```python
from build123d import *


with BuildPart() as part:
    # Sweep5: sweep along a path in Sketch1
    with BuildLine(Plane.XY) as sweep5_path:
        Line((0, 0), (0, 450))
        ThreePointArc((0, 450), (14.644660941, 485.355339059), (50, 500))
        Line((50, 500), (450, 500))
        ThreePointArc((450, 500), (485.355339059, 514.644660941), (500, 550))
        Line((500, 550), (500, 1000))
    # Sketch12 → Sweep5 (sweep)
    with BuildSketch(Plane(origin=(0, 0, 0), x_dir=(1, 0, 0), z_dir=(0, 1, 0))):
        Polygon((-14.43375673, -25), (14.43375673, -25), (28.867513459, 0), (14.43375673, 25), (-14.43375673, 25), (-28.867513459, 0), align=None)
    sweep(path=sweep5_path.line)


solid = part.part
```
Geometry check sheet. Reference: the model listing, model coordinates, mm. A direction names the side the tool comes from. Coordinates: 2 decimals unless noted, no trailing zeros. Order: outer loops, then holes, each group sorted by start corner. A loop starts at its lowest first (then second) coordinate and runs counter-clockwise, first axis right, second up.
Q1. Sectioned sample at B-B on z = -15. Record the cut outline in (x, y), and give its area (3 significant figures).
Reply:
outline: (-20.21, 0) - (20.21, 0) - (20.21, 450) arc R29.79 cw to (50, 479.79) - (450, 479.79) arc R70.21 ccw to (520.21, 550) - (520.21, 1000) - (479.79, 1000) - (479.79, 550) arc R29.79 cw to (450, 520.21) - (50, 520.21) arc R70.21 ccw to (-20.21, 450) - close
area: 58,900 mm2
Q2. Thickness scan on probe 1 along X at (y, z) = (442, 0); probe 2 along X at (y, z) = (229.5, 14.5); probe 3 along Y at (x, z) = (189.5, -14). Record the ranges inside material, lowest first.
Reply:
probe 1: x = -28.87 to 28.87
probe 2: x = -20.5 to 20.5
probe 3: y = 479.22 to 520.78
Q3. Tool access check on faces 1 (the face through (478.25, 778.15, 12.33)), 2 (the face through (478.45, 778.15, -12.675)), 3 (the face through (-21.75, 228.15, 12.33)), 4 (the face through (252.8, 478.45, 12.675)). Record the directions out of +Z, -Z, +X, -X, +Y, -Y that give a thin tool (end or side, any length) a straight path to the whole face; none if there is none.
Reply:
face 1: +Z, -X, +Y
face 2: -Z, -X, +Y
face 3: +Z, -X, +Y, -Y
face 4: +Z, +X, -Y
Q4. Sectioned sample at A-A on x = 157. Record the cut outline in (y, z).
Reply:
outline: (471.13, 0) - (485.57, -25) - (514.43, -25) - (528.87, 0) - (514.43, 25) - (485.57, 25) - close
Q5. Sectioned sample at C-C on y = 229.5. Record the cut outline in (x, z).
Reply:
outline: (-28.87, 0) - (-14.43, -25) - (14.43, -25) - (28.87, 0) - (14.43, 25) - (-14.43, 25) - close
Q6. Depth check by flat-ended pin: pin 1 Ø5 at (y, z) = (696.5, -19.5) entering from +X; pin 2 Ø3 at (y, z) = (826, 16.5) entering from -X; pin 3 Ø1 at (y, z) = (121, 17) entering from -X. Enter the tip coordinate at first touch or a pass-through.
Reply:
pin 1: stops at x = 519.05
pin 2: stops at x = 479.79
pin 3: stops at x = -19.34
